Part model, mm, in its own coordinate system. Round coordinates to 2 decimals unless told otherwise and drop trailing zeros. Loops run counter-clockwise (first coordinate to the right, second up) from the corner with the lowest first, then second, coordinate; pieces in that order, holes last. Notation, with made-up numbers: M -40,2.5 L -28,2.5 A31 cw -28,41.5 Z; hole C 6,41.25 d2. An arc over 180 degrees is marked long. Put each result on its own line as item: value. Start each with the question number.
1) Probe line 1 along Z through (x, y) = (0, -0.65); line 2 along X through (y, z) = (-1.4, -16); line 3 along X through (y, z) = (-1.35, -14.5). List the from-to ranges inside material, lowest first.
2) Slice it at D-D on x = 16.5. Give the cut face in (y, z).
3) Slice it at A-A on x = 0. Give the cut face in (y, z).
4) Drop a flat-ended pin along its axis: pin 1 Ø1.9 at (x, z) = (-15.5, 15.5) entering from -Y. Give the stop position or say it passes through.
5) Slice it at C-C on y = -1.2. State how many separate pieces and enclosed holes the cut face has, then the cut area to 3 significant figures.
6) Slice it at B-B on z = 6. Give the cut face in (x, y), then the cut area to 3 significant figures.
```python
from build123d import *

# Parameters (mm, degrees)
F0_W     = 45
F0_H     = 45
F0_R     = 1.6
F0_R_2   = 11.05
F1_DEPTH = 2


with BuildPart() as f1:
    # F0 (on Front) → F1 (new body)
    with BuildSketch(Plane.XZ):
        Rectangle(F0_W, F0_H)
        with Locations((-15.5, -15.5)):
            Circle(F0_R, mode=Mode.SUBTRACT)
        with Locations((15.5, -15.5)):
            Circle(F0_R, mode=Mode.SUBTRACT)
        with Locations((-15.5, 15.5)):
            Circle(F0_R, mode=Mode.SUBTRACT)
        with BuildLine():
            ThreePointArc((10.964367, 8.705323), (12.934313, 5.357568), (13.908571, 1.597386))
            ThreePointArc((13.908571, 1.597386), (15.09857, 1.163247), (15.6, 0))
            ThreePointArc((15.6, 0), (15.09857, -1.163247), (13.908571, -1.597386))
            ThreePointArc((13.908571, -1.597386), (12.934313, -5.357568), (10.964367, -8.705323))
            ThreePointArc((10.964367, -8.705323), (11.359597, -9.2452), (11.499495, -9.899495))
            ThreePointArc((11.499495, -9.899495), (10.469287, -11.394599), (8.705323, -10.964367))
            ThreePointArc((8.705323, -10.964367), (5.357568, -12.934313), (1.597386, -13.908571))
            ThreePointArc((1.597386, -13.908571), (1.599346, -13.954267), (1.6, -14))
            ThreePointArc((1.6, -14), (-0.045733, -15.599346), (-1.597386, -13.908571))
            ThreePointArc((-1.597386, -13.908571), (-5.357568, -12.934313), (-8.705323, -10.964367))
            ThreePointArc((-8.705323, -10.964367), (-11.030866, -11.030866), (-10.964367, -8.705323))
            ThreePointArc((-10.964367, -8.705323), (-12.934313, -5.357568), (-13.908571, -1.597386))
            ThreePointArc((-13.908571, -1.597386), (-15.6, 0), (-13.908571, 1.597386))
            ThreePointArc((-13.908571, 1.597386), (-12.934313, 5.357568), (-10.964367, 8.705323))
            ThreePointArc((-10.964367, 8.705323), (-11.030866, 11.030866), (-8.705323, 10.964367))
            ThreePointArc((-8.705323, 10.964367), (-5.357568, 12.934313), (-1.597386, 13.908571))
            ThreePointArc((-1.597386, 13.908571), (-0.045733, 15.599346), (1.6, 14))
            ThreePointArc((1.6, 14), (1.599346, 13.954267), (1.597386, 13.908571))
            ThreePointArc((1.597386, 13.908571), (5.357568, 12.934313), (8.705323, 10.964367))
            ThreePointArc((8.705323, 10.964367), (10.469287, 11.394599), (11.499495, 9.899495))
            ThreePointArc((11.499495, 9.899495), (11.359597, 9.2452), (10.964367, 8.705323))
        make_face(mode=Mode.SUBTRACT)
        with Locations((15.5, 15.5)):
            Circle(F0_R, mode=Mode.SUBTRACT)
        with BuildLine():
            ThreePointArc((13.908571, -1.597386), (12.4, 0), (13.908571, 1.597386))
            ThreePointArc((13.908571, 1.597386), (12.934313, 5.357568), (10.964367, 8.705323))
            ThreePointArc((10.964367, 8.705323), (8.768124, 8.768124), (8.705323, 10.964367))
            ThreePointArc((8.705323, 10.964367), (5.357568, 12.934313), (1.597386, 13.908571))
            ThreePointArc((1.597386, 13.908571), (0, 12.4), (-1.597386, 13.908571))
            ThreePointArc((-1.597386, 13.908571), (-5.357568, 12.934313), (-8.705323, 10.964367))
            ThreePointArc((-8.705323, 10.964367), (-8.40439, 10.469287), (-8.299495, 9.899495))
            ThreePointArc((-8.299495, 9.899495), (-9.2452, 8.439393), (-10.964367, 8.705323))
            ThreePointArc((-10.964367, 8.705323), (-12.934313, 5.357568), (-13.908571, 1.597386))
            ThreePointArc((-13.908571, 1.597386), (-12.836753, 1.09857), (-12.4, 0))
            ThreePointArc((-12.4, 0), (-12.836753, -1.09857), (-13.908571, -1.597386))
            ThreePointArc((-13.908571, -1.597386), (-12.934313, -5.357568), (-10.964367, -8.705323))
            ThreePointArc((-10.964367, -8.705323), (-9.2452, -8.439393), (-8.299495, -9.899495))
            ThreePointArc((-8.299495, -9.899495), (-8.40439, -10.469287), (-8.705323, -10.964367))
            ThreePointArc((-8.705323, -10.964367), (-5.357568, -12.934313), (-1.597386, -13.908571))
            ThreePointArc((-1.597386, -13.908571), (0, -12.4), (1.597386, -13.908571))
            ThreePointArc((1.597386, -13.908571), (5.357568, -12.934313), (8.705323, -10.964367))
            ThreePointArc((8.705323, -10.964367), (8.768124, -8.768124), (10.964367, -8.705323))
            ThreePointArc((10.964367, -8.705323), (12.934313, -5.357568), (13.908571, -1.597386))
        make_face()
        Circle(F0_R_2, mode=Mode.SUBTRACT)
    extrude(amount=F1_DEPTH)


solid = f1.part
```
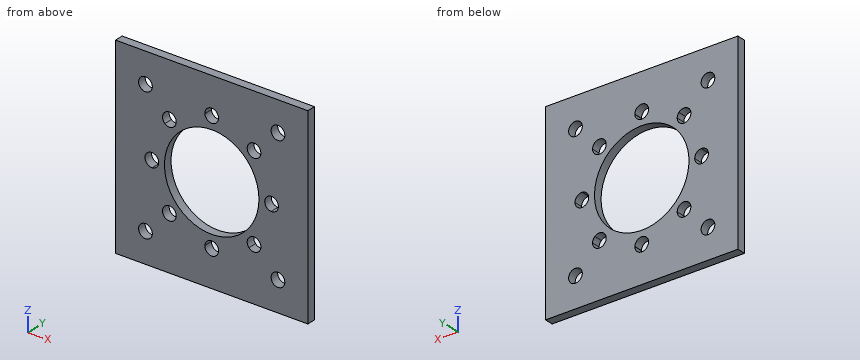
Recorded:
1. line 1: z = -22.5 to -15.6, -12.4 to -11.05, 11.05 to 12.4, 15.6 to 22.5
1. line 2: x = -22.5 to -17.02, -13.98 to 13.98, 17.02 to 22.5
1. line 3: x = -22.5 to -16.75, -14.25 to -1.52, 1.52 to 14.25, 16.75 to 22.5
2. outline: M -2,-22.5 L 0,-22.5 L 0,-16.75 L -2,-16.75 Z; M -2,-14.25 L 0,-14.25 L 0,14.25 L -2,14.25 Z; M -2,16.75 L 0,16.75 L 0,22.5 L -2,22.5 Z
3. outline: M -2,-22.5 L 0,-22.5 L 0,-15.6 L -2,-15.6 Z; M -2,-12.4 L 0,-12.4 L 0,-11.05 L -2,-11.05 Z; M -2,11.05 L 0,11.05 L 0,12.4 L -2,12.4 Z; M -2,15.6 L 0,15.6 L 0,22.5 L -2,22.5 Z
4. pin 1: passes through
5. separate pieces: 1
5. enclosed holes: 13
5. area: 1,540 mm2
6. outline: M -22.5,-2 L -9.28,-2 L -9.28,0 L -22.5,0 Z; M 9.28,-2 L 22.5,-2 L 22.5,0 L 9.28,0 Z
6. area: 52.9 mm2
